Design review of the part shown in the three views and the two pictorial views. Dimensions are in mm from the part's minimum x, y and z. Coordinates: 2 decimals unless noted, no trailing zeros. Order: outer loops, then holes, each group sorted by start corner. A loop starts at its lowest first (then second) coordinate and runs counter-clockwise, first axis right, second up. Notation, with made-up numbers: (-15, 84) -> (18, 84) arc R10 cw to (18, 100) -> close; hole circle Ø4 at (-7, 40). An arc over 180 degrees is marked (long way). Write item = value, one per line. Start each with the question number.
1) Insertion check: pin 1 Ø4 at (x, y) = (14, 10) entering from +Z. The pin has a flat end and moves straight along its axis. Give the tip position at first contact, or say it passes through.
2) Draft analysis for pull direction X (two halves, no side actions). For the marked faces 1, 2 and 3, state which applies: +X half, -X half, draft (parallel to the pull), parting line (faces both ways), or undercut.
3) Consider section A-A on y = 8.5. Give the boundary of the cut face in (x, z), and give its area (3 significant figures).
4) Wall thickness on probe 1 along Y at (x, z) = (7.25, 2.3): over which ranges is the line inside the solid? List them lowest first. Write a range as [from, to].
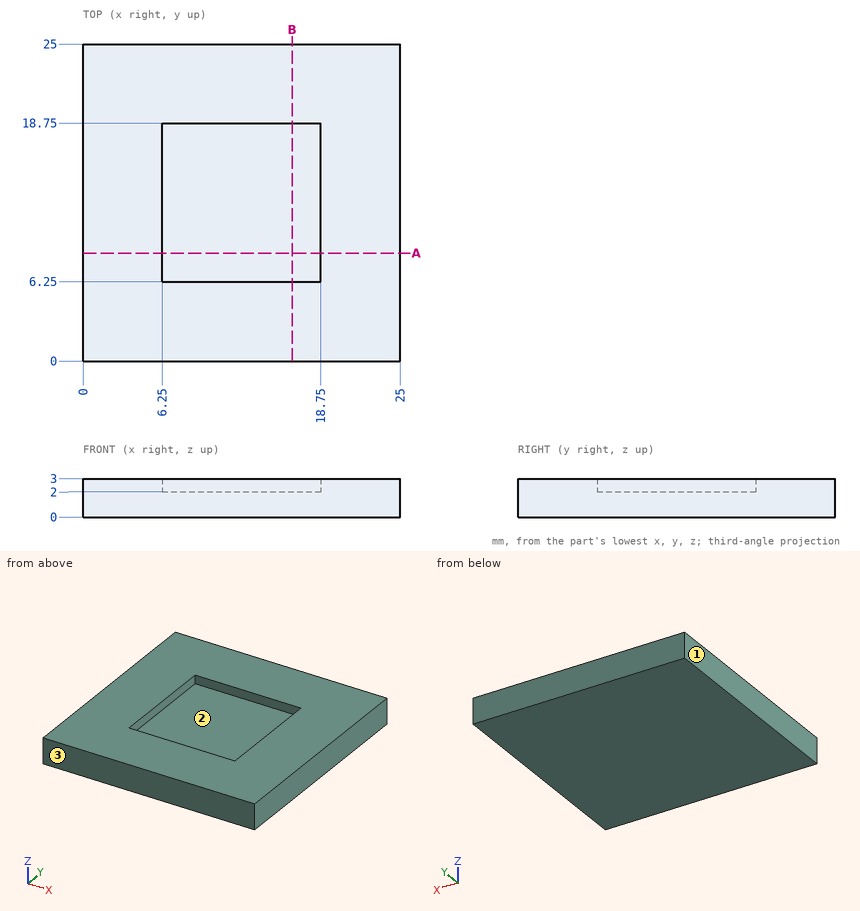
Answer sheet:
q1.pin_1 = 2
q2.face_1 = -X half
q2.face_2 = undercut
q2.face_3 = draft
q3.outline = (0, 0) -> (25, 0) -> (25, 3) -> (18.75, 3) -> (18.75, 2) -> (6.25, 2) -> (6.25, 3) -> (0, 3) -> close
q3.area = 62.5 mm2
q4.probe_1 = [0, 6.25], [18.75, 25]
